from build123d import *

# Parameters (mm, degrees)
SKETCH1_W                               = 125
SKETCH1_H                               = 90
BOSS_EXTRUDE1_DEPTH                     = 40
FILLET1_R                               = 6
CBORE_FOR_M5_HEX_HEAD_BOLT1_D           = 3
CBORE_FOR_M5_HEX_HEAD_BOLT1_DEPTH       = 12
CBORE_FOR_M5_HEX_HEAD_BOLT1_CBORE_D     = 4.2
CBORE_FOR_M5_HEX_HEAD_BOLT1_CBORE_DEPTH = 5
CBORE_FOR_M5_HEX_HEAD_BOLT1_TIP         = 0.901290929
SHELL2_START                            = 4
SHELL2_DEPTH                            = 36
SHELL2_2_DEPTH                          = 21.736908887
SHELL2_START_2                          = 23.633896721
SHELL2_3_DEPTH                          = 7.366103279
SKETCH11_W                              = 95
SKETCH11_H                              = 36
CUT_EXTRUDE4_DEPTH                      = 117.645831473
SKETCH12_W                              = 36
SKETCH12_H                              = 60
CUT_EXTRUDE5_DEPTH                      = 139.744369255
SKETCH7_R                               = 3
BOSS_EXTRUDE2_DEPTH                     = 5
M3X0_5_TAPPED_HOLE1_D                   = 2.5
M3X0_5_TAPPED_HOLE1_DEPTH               = 7.5
M3X0_5_TAPPED_HOLE1_TIP                 = 0.751075774
FILLET3_R                               = 18
FILLET4_R                               = 18
CUT_EXTRUDE1_DEPTH                      = 86.013234264
SKETCH7_5_R                             = 5
CUT_EXTRUDE2_DEPTH                      = 86.013234264
CUT_EXTRUDE3_DEPTH                      = 86.013234264


with BuildPart() as part:
    # Sketch1 → Boss-Extrude1 (new body)
    with BuildSketch(Plane.XY):
        Rectangle(SKETCH1_W, SKETCH1_H)
    extrude(amount=BOSS_EXTRUDE1_DEPTH)

    # Fillet1
    fillet1_edges = [part.edges().sort_by_distance(p)[0] for p in [
        (62.5, -45, 20),
        (-62.5, -45, 20),
        (-62.5, 45, 20),
        (62.5, 45, 20),
    ]]
    fillet(fillet1_edges, radius=FILLET1_R)

    # CBORE for M5 Hex Head Bolt1
    with Locations(Plane.XY.offset(40)):
        with Locations((-56.5, 39), (56.5, 39), (56.5, -39), (-56.5, -39)):
            CounterBoreHole(CBORE_FOR_M5_HEX_HEAD_BOLT1_D / 2, CBORE_FOR_M5_HEX_HEAD_BOLT1_CBORE_D / 2, CBORE_FOR_M5_HEX_HEAD_BOLT1_CBORE_DEPTH, depth=CBORE_FOR_M5_HEX_HEAD_BOLT1_DEPTH)
            with Locations((0, 0, -(CBORE_FOR_M5_HEX_HEAD_BOLT1_DEPTH + CBORE_FOR_M5_HEX_HEAD_BOLT1_TIP / 2))):  # 118° drill point
                Cone(0, CBORE_FOR_M5_HEX_HEAD_BOLT1_D / 2, CBORE_FOR_M5_HEX_HEAD_BOLT1_TIP, mode=Mode.SUBTRACT)

    # Shell2: read off the stored shape, not the designer's step
    # Shell2 outline → Shell2 (cut)
    with BuildSketch(Plane.XY.offset(SHELL2_START)):
        with BuildLine():
            ThreePointArc((58.5, 33.237188186), (52.186648635, 34.686648635), (50.737188186, 41))
            Line((50.737188186, 41), (-50.737188186, 41))
            ThreePointArc((-50.737188186, 41), (-52.186648635, 34.686648635), (-58.5, 33.237188186))
            Line((-58.5, 33.237188186), (-58.5, -33.237188186))
            ThreePointArc((-58.5, -33.237188186), (-52.186648635, -34.686648635), (-50.737188186, -41))
            Line((-50.737188186, -41), (50.737188186, -41))
            ThreePointArc((50.737188186, -41), (52.186648635, -34.686648635), (58.5, -33.237188186))
            Line((58.5, -33.237188186), (58.5, 33.237188186))
        make_face()
    extrude(amount=SHELL2_DEPTH, mode=Mode.SUBTRACT)

    # Shell2 2 outline → Shell2 2 (cut)
    with BuildSketch(Plane.XY.offset(SHELL2_START)):
        with BuildLine():
            Line((56.5, 41), (50.737188186, 41))
            ThreePointArc((50.737188186, 41), (52.186648635, 34.686648635), (58.5, 33.237188186))
            Line((58.5, 33.237188186), (58.5, 39))
            ThreePointArc((58.5, 39), (57.914213562, 40.414213562), (56.5, 41))
        make_face()
        with BuildLine():
            ThreePointArc((-58.5, 33.237188186), (-52.186648635, 34.686648635), (-50.737188186, 41))
            Line((-50.737188186, 41), (-56.5, 41))
            ThreePointArc((-56.5, 41), (-57.914213562, 40.414213562), (-58.5, 39))
            Line((-58.5, 39), (-58.5, 33.237188186))
        make_face()
        with BuildLine():
            ThreePointArc((58.5, -33.237188186), (52.186648635, -34.686648635), (50.737188186, -41))
            Line((50.737188186, -41), (56.5, -41))
            ThreePointArc((56.5, -41), (57.914213562, -40.414213562), (58.5, -39))
            Line((58.5, -39), (58.5, -33.237188186))
        make_face()
        with BuildLine():
            ThreePointArc((-50.737188186, -41), (-52.186648635, -34.686648635), (-58.5, -33.237188186))
            Line((-58.5, -33.237188186), (-58.5, -39))
            ThreePointArc((-58.5, -39), (-57.914213562, -40.414213562), (-56.5, -41))
            Line((-56.5, -41), (-50.737188186, -41))
        make_face()
    extrude(amount=SHELL2_2_DEPTH, mode=Mode.SUBTRACT)

    # Shell2 3 outline → Shell2 3 (cut)
    with BuildSketch(Plane.XY.offset(SHELL2_START_2)):
        with BuildLine():
            ThreePointArc((58.5, 33.876524617), (52.610912703, 35.110912703), (51.376524617, 41))
            Line((51.376524617, 41), (50.737188186, 41))
            ThreePointArc((50.737188186, 41), (52.186648635, 34.686648635), (58.5, 33.237188186))
            Line((58.5, 33.237188186), (58.5, 33.876524617))
        make_face()
        with BuildLine():
            ThreePointArc((-58.5, 33.237188186), (-52.186648635, 34.686648635), (-50.737188186, 41))
            Line((-50.737188186, 41), (-51.376524617, 41))
            ThreePointArc((-51.376524617, 41), (-52.610912703, 35.110912703), (-58.5, 33.876524617))
            Line((-58.5, 33.876524617), (-58.5, 33.237188186))
        make_face()
        with BuildLine():
            Line((58.5, -33.876524617), (58.5, -33.237188186))
            ThreePointArc((58.5, -33.237188186), (52.186648635, -34.686648635), (50.737188186, -41))
            Line((50.737188186, -41), (51.376524617, -41))
            ThreePointArc((51.376524617, -41), (52.610912703, -35.110912703), (58.5, -33.876524617))
        make_face()
        with BuildLine():
            ThreePointArc((-50.737188186, -41), (-52.186648635, -34.686648635), (-58.5, -33.237188186))
            Line((-58.5, -33.237188186), (-58.5, -33.876524617))
            ThreePointArc((-58.5, -33.876524617), (-52.610912703, -35.110912703), (-51.376524617, -41))
            Line((-51.376524617, -41), (-50.737188186, -41))
        make_face()
    extrude(amount=SHELL2_3_DEPTH, mode=Mode.SUBTRACT)

    # Shell2 4 outline → Shell2 4 (revolve)
    with BuildSketch(Plane(origin=(56.5, 39, 0), x_dir=(1, 0, 0), z_dir=(0, -1, 0))):
        Polygon((0, 25.736908889), (0, 22.432175483), (5.500000002, 25.736908889), align=None)
    revolve(axis=Axis((56.5, 39, 0), (0, 0, 1)))

    # Shell2 5 outline → Shell2 5 (revolve)
    with BuildSketch(Plane(origin=(56.5, -39, 0), x_dir=(1, 0, 0), z_dir=(0, -1, 0))):
        Polygon((0, 25.736908889), (0, 22.432175483), (5.500000002, 25.736908889), align=None)
    revolve(axis=Axis((56.5, -39, 0), (0, 0, 1)))

    # Shell2 6 outline → Shell2 6 (revolve)
    with BuildSketch(Plane(origin=(-56.5, 39, 0), x_dir=(1, 0, 0), z_dir=(0, -1, 0))):
        Polygon((0, 25.736908889), (0, 22.432175483), (5.500000002, 25.736908889), align=None)
    revolve(axis=Axis((-56.5, 39, 0), (0, 0, 1)))

    # Shell2 7 outline → Shell2 7 (revolve)
    with BuildSketch(Plane(origin=(-56.5, -39, 0), x_dir=(1, 0, 0), z_dir=(0, -1, 0))):
        Polygon((0, 25.736908887), (0, 22.432175483), (5.5, 25.736908887), align=None)
    revolve(axis=Axis((-56.5, -39, 0), (0, 0, 1)))

    # Sketch11 → Cut-Extrude4 (cut, through all)
    with BuildSketch(Plane.XZ.offset(45)):
        with Locations((0, 22)):
            Rectangle(SKETCH11_W, SKETCH11_H)
    extrude(amount=-CUT_EXTRUDE4_DEPTH, mode=Mode.SUBTRACT)

    # Sketch12 → Cut-Extrude5 (cut, through all)
    with BuildSketch(Plane(origin=(62.5, 0, 0), x_dir=(0, 0, -1), z_dir=(1, 0, 0))):
        with Locations((-22, 0)):
            Rectangle(SKETCH12_W, SKETCH12_H)
    extrude(amount=-CUT_EXTRUDE5_DEPTH, mode=Mode.SUBTRACT)

    # Sketch7 → Boss-Extrude2 (add)
    with BuildSketch(Plane.XY.offset(4)):
        with Locations((-52.15, 27.94)):
            Circle(SKETCH7_R)
        with Locations((-21.67, 27.94)):
            Circle(SKETCH7_R)
        with Locations((-52.15, -27.94)):
            Circle(SKETCH7_R)
        with Locations((-21.67, -27.94)):
            Circle(SKETCH7_R)
    extrude(amount=BOSS_EXTRUDE2_DEPTH)

    # M3x0.5 Tapped Hole1
    with Locations(Plane.XY.offset(9)):
        with Locations((-52.15, 27.94), (-21.67, 27.94), (-21.67, -27.94), (-52.15, -27.94)):
            Hole(M3X0_5_TAPPED_HOLE1_D / 2, depth=M3X0_5_TAPPED_HOLE1_DEPTH)
            with Locations((0, 0, -(M3X0_5_TAPPED_HOLE1_DEPTH + M3X0_5_TAPPED_HOLE1_TIP / 2))):  # 118° drill point
                Cone(0, M3X0_5_TAPPED_HOLE1_D / 2, M3X0_5_TAPPED_HOLE1_TIP, mode=Mode.SUBTRACT)

    # Fillet3
    fillet3_edges = [part.edges().sort_by_distance(p)[0] for p in [
        (47.5, 43, 4),
        (-47.5, 43, 4),
        (47.5, -43, 4),
        (-47.5, -43, 4),
    ]]
    fillet(fillet3_edges, radius=FILLET3_R)

    # Fillet4
    fillet4_edges = [part.edges().sort_by_distance(p)[0] for p in [
        (60.5, 30, 4),
        (60.5, -30, 4),
        (-60.5, 30, 4),
        (-60.5, -30, 4),
    ]]
    fillet(fillet4_edges, radius=FILLET4_R)

    # Sketch7<4> → Cut-Extrude1 (cut, through all)
    with BuildSketch(Plane.XY.offset(4)):
        with BuildLine():
            Line((-52.15, 1.75), (-46.15, 1.75))
            ThreePointArc((-46.15, 1.75), (-44.4, 0), (-46.15, -1.75))
            Line((-46.15, -1.75), (-52.15, -1.75))
            ThreePointArc((-52.15, -1.75), (-53.9, 0), (-52.15, 1.75))
        make_face()
    extrude(amount=-CUT_EXTRUDE1_DEPTH, mode=Mode.SUBTRACT)

    # Sketch7<5> → Cut-Extrude2 (cut, through all)
    with BuildSketch(Plane.XY.offset(4)):
        with Locations((0, -27.94)):
            Circle(SKETCH7_5_R)
    extrude(amount=-CUT_EXTRUDE2_DEPTH, mode=Mode.SUBTRACT)

    # Sketch7<6> → Cut-Extrude3 (cut, through all)
    with BuildSketch(Plane.XY.offset(4)):
        with BuildLine():
            Line((53.9, 3), (53.9, -3))
            ThreePointArc((53.9, -3), (52.15, -4.75), (50.4, -3))
            Line((50.4, -3), (50.4, 3))
            ThreePointArc((50.4, 3), (52.15, 4.75), (53.9, 3))
        make_face()
    extrude(amount=-CUT_EXTRUDE3_DEPTH, mode=Mode.SUBTRACT)


solid = part.part
For this review, take the finished solid that the model builds, in its own axes (mm). A direction names the side the tool comes from. Give positions to 0.01 mm unless a question says otherwise; leave off trailing zeros. Order: outer loops, then holes, each group sorted by start corner. A loop starts at its lowest first (then second) coordinate and runs counter-clockwise, first axis right, second up. Notation, with made-up numbers: (-38, 52) -> (18, 52) arc R11 cw to (18, 68) -> close; hole circle Ø2 at (7.5, 51). An arc over 180 degrees is marked (long way). Write item = value, one per line.
1) Draft analysis for pull direction X (two halves, no side actions). For faces 1 (the face through (52.255, 34.62, 35.437)), 2 (the face through (-60.528, 24.867, 9.413)), 3 (the face through (-60.789, -43.196, 20.28)), 4 (the face through (-53.34, -27.56, 5.2)), state which applies: pulls with the +X half, pulls with the -X half, needs draft (parallel to the pull), parting line crosses it, or undercut.
Findings:
face_1 = undercut
face_2 = needs draft
face_3 = pulls with the -X half
face_4 = undercut
2) We need section A-A, the plane y = 0. Give the boundary of the cut face in (x, z).
Findings:
outline = (-62.5, 0) -> (-53.9, 0) -> (-53.9, 4) -> (-62.5, 4) -> close; (-44.4, 0) -> (50.4, 0) -> (50.4, 4) -> (-44.4, 4) -> close; (53.9, 0) -> (62.5, 0) -> (62.5, 4) -> (53.9, 4) -> close
3) We need section B-B, the plane x = 0. Give the boundary of the cut face in (y, z), and give its area (3 significant figures).
Findings:
outline = (-45, 0) -> (-32.94, 0) -> (-32.94, 4) -> (-45, 4) -> close; (-22.94, 0) -> (45, 0) -> (45, 4) -> (-22.94, 4) -> close
area = 320 mm^2
4) We need section C-C, the plane z = 18. Count the separate pieces of the cut face and the enclosed holes in it, and give its area (3 significant figures).
Findings:
separate_pieces = 4
enclosed_holes = 0
area = 403 mm^2
5) For faces 5 (the face through (47.5, -43, 31)), 6 (the face through (-60, -30, 31)), 7 (the face through (-22.825, -28.419, 5.198)), list the 3-axis set-ups (+Z, -Z, +X, -X, +Y, -Y) from which the entire face can be reached by the end or side of a thin tool; tool diameter is ignored.
Findings:
face_5 = +Z, +Y, -Y
face_6 = +Z, +X, -X
face_7 = +Z
6) To check wall thickness, follow L1, parallel to Y at x = 56, z = 5; L2, parallel to X at y = 39, z = 14; L3, parallel to Z at x = -48.5, y = 38. State the ranges of each line that lie inside material, in increasing order. Write a range as from..to.
Findings:
L1 = -45..-41, 41..45
L2 = -62.5..-58.5, 58.5..62.5
L3 = 0..4
7) Insertion check: pin 1 (1.8 mm diameter, centred on x = 56.5, y = 39, fed in from +Z); pin 2 (5 mm diameter, centred on x = -21, z = 13, fed in from +Y); pin 3 (2.5 mm diameter, centred on x = -56.5, y = 39, fed in from -Z); pin 4 (4.5 mm diameter, centred on x = 60.5, z = 34.5, fed in from +Y). Each pin has a flat end and moves straight along its axis. Give the tip position at first contact, or say it passes through.
Findings:
pin_1 = 27.64
pin_2 = through
pin_3 = 0
pin_4 = 44.74
